```python
from build123d import *

# Parameters (mm, degrees)
F0_R     = 102.785
F0_R_2   = 99.8
F1_DEPTH = 55
F2_DEPTH = 108
F3_SIZE  = 5


with BuildPart() as f1:
    # F0 (on Front) → F1 (new body)
    with BuildSketch(Plane.XZ):
        Circle(F0_R)
        Circle(F0_R_2, mode=Mode.SUBTRACT)
    extrude(amount=F1_DEPTH)

    # F0 (on Front) → F2 (join)
    with BuildSketch(Plane.XZ):
        Circle(F0_R_2)
    extrude(amount=F2_DEPTH)

    # F3
    f3_edges = [f1.edges().sort_by_distance(p)[0] for p in [
        (-99.8, -108, 0),
    ]]
    chamfer(f3_edges, length=F3_SIZE)


solid = f1.part
```
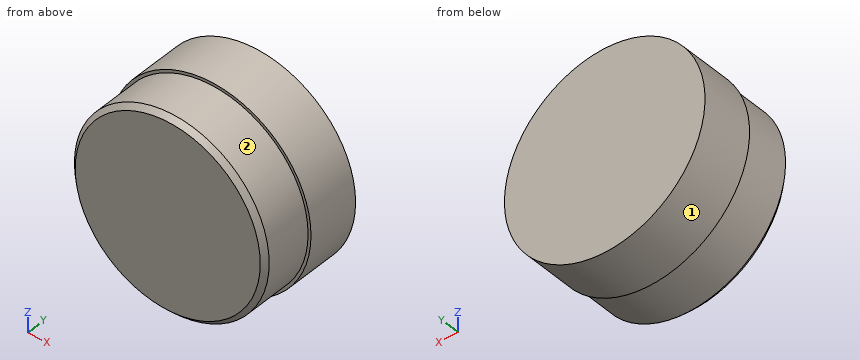
Input: part model. Units: mm. Frame: model coordinates. Face numbers are marked on the shaded views. A direction names the side the tool comes from. Round coordinates to 2 decimals unless told otherwise and drop trailing zeros. Loops run counter-clockwise (first coordinate to the right, second up) from the corner with the lowest first, then second, coordinate; pieces in that order, holes last. Notation, with made-up numbers: M 63,-31 L 73,-31 A24 cw 73,0 Z; hole C -34.5,22.5 d2. An arc over 180 degrees is marked long. Answer in a Markdown table with one row per item. Add a question column.
1. Section A-A (z = 0). Output: boundary loops of the cut face in (x, y) (3 decimals).
2. Ray query, probe 1 along X at (y, z) = (-103, -1); probe 2 along X at (y, z) = (-100, 48); probe 3 along Z at (x, y) = (-9.5, -75). Return the intervals inside material, ascending.
3. Section B-B (x = 0). Output: boundary loops of the cut face in (y, z) (3 decimals), and give its area (3 significant figures).
4. Contact query for flat-ended pins moving along their axis: pin 1 (8 mm diameter, centred on y = -80.5, z = 61, fed in from -X); pin 2 (6 mm diameter, centred on x = 32, y = -74.5, fed in from +Z); pin 3 (3 mm diameter, centred on x = -16.5, y = -69.5, fed in from +Z). Output: stop coordinate, or through.
5. Section C-C (y = -93). Output: boundary loops of the cut face in (x, z), and give its area (3 significant figures).
6. Section D-D (y = -11.5). Output: boundary loops of the cut face in (x, z) (3 decimals).
7. Set-up query: the marked faces 1 and 2. Return all of +Z, -Z, +X, -X, +Y, -Y with unobstructed straight access to the full face (end or side cutting, diameter ignored); none if empty.
Values follow:
| question | item | result |
|---|---|---|
| 1 | outline | M -102.785,-55 L -99.8,-55 L -99.8,-103 L -94.8,-108 L 94.8,-108 L 99.8,-103 L 99.8,-55 L 102.785,-55 L 102.785,0 L -102.785,0 Z |
| 2 | probe 1 | -99.79 to 99.79 |
| 2 | probe 2 | -87.5 to 87.5 |
| 2 | probe 3 | -99.35 to 99.35 |
| 3 | outline | M -108,-94.8 L -103,-99.8 L -55,-99.8 L -55,-102.785 L 0,-102.785 L 0,102.785 L -55,102.785 L -55,99.8 L -103,99.8 L -108,94.8 Z |
| 3 | area | 21,900 mm^2 |
| 4 | pin 1 | x = -81.92 |
| 4 | pin 2 | z = 95.49 |
| 4 | pin 3 | z = 98.67 |
| 5 | outline | C 0,0 d199.6 |
| 5 | area | 31,300 mm^2 |
| 6 | outline | C 0,0 d205.57 |
| 7 | face 1 | +Y, -Y |
| 7 | face 2 | -Y |
